Model file for the job. Use its own axes, mm. Face numbers are marked on the shaded views. Give positions to 0.01 mm unless a question says otherwise; leave off trailing zeros. Write each loop counter-clockwise with the first axis right and the second up, starting at its lowest first coordinate (ties: lowest second). Pieces come first, ordered by that corner, then holes. Notation, with made-up numbers: (39.5, -28) - (85.5, -28) arc R32 cw to (85.5, 11) - close; hole circle Ø4 at (20, 45). An arc over 180 degrees is marked (long way). One line per item, written item: value. Start each with the question number.
(1) Drop a flat-ended pin along its axis: P1, Ø4, axis at x = -4, z = 1, coming from the +Y side. Give the stop position or say it passes through.
(2) Cut at A-A, the plane y = 38. List the corners of the cut face in (x, z), and give its area (3 significant figures).
(3) Cut at C-C, the plane x = -8.25. List the corners of the cut face in (y, z).
(4) Cut at B-B, the plane z = -2. List the corners of the cut face in (x, y), and give its area (3 significant figures).
(5) Cut at D-D, the plane y = 8.5. List the corners of the cut face in (x, z), and give its area (3 significant figures).
(6) Mould opens along X. For the marked faces 1, 2 and 3 say: pulls with the +X half, pulls with the -X half, needs draft (parallel to the pull), parting line crosses it, or undercut.
(7) Probe L1, parallel to Z at x = -0.25, y = 20; L2, parallel to X at y = 19, z = -0.5; L3, parallel to X at y = 9, z = -2. List the from-to ranges inside material, lowest first.
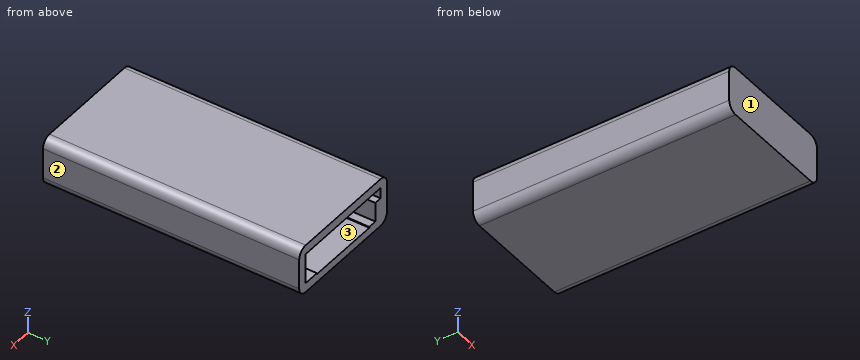
from build123d import *

# Parameters (mm, degrees)
SKETCH1_W           = 20.3
SKETCH1_H           = 7.9
SKETCH1_W_2         = 17.3
SKETCH1_H_2         = 4.9
BOSS_EXTRUDE1_DEPTH = 41.5
SKETCH2_W           = 20.3
SKETCH2_H           = 7.9
BOSS_EXTRUDE2_DEPTH = 1.5
SKETCH3_W           = 1.2
SKETCH3_H           = 3.15
BOSS_EXTRUDE3_DEPTH = 40
SKETCH4_W           = 1.2
SKETCH4_H           = 3.15
BOSS_EXTRUDE4_DEPTH = 17
SKETCH5_W           = 12.1
SKETCH5_H           = 0.3
CUT_EXTRUDE1_DEPTH  = 4.3
FILLET1_R           = 1.5


with BuildPart() as part:
    # Sketch1 → Boss-Extrude1 (new body)
    with BuildSketch(Plane(origin=(0, 0, 0), x_dir=(1, 0, 0), z_dir=(0, 1, 0))):
        Rectangle(SKETCH1_W, SKETCH1_H)
        Rectangle(SKETCH1_W_2, SKETCH1_H_2, mode=Mode.SUBTRACT)
    extrude(amount=BOSS_EXTRUDE1_DEPTH)

    # Sketch2 → Boss-Extrude2 (add)
    with BuildSketch(Plane.XZ):
        Rectangle(SKETCH2_W, SKETCH2_H)
    extrude(amount=-BOSS_EXTRUDE2_DEPTH)

    # Sketch3 → Boss-Extrude3 (add)
    with BuildSketch(Plane(origin=(0, 1.5, 0), x_dir=(1, 0, 0), z_dir=(0, 1, 0))):
        with Locations((-8.05, 0.875)):
            Rectangle(SKETCH3_W, SKETCH3_H)
    extrude(amount=BOSS_EXTRUDE3_DEPTH)

    # Sketch4 → Boss-Extrude4 (add)
    with BuildSketch(Plane(origin=(0, 1.5, 0), x_dir=(1, 0, 0), z_dir=(0, 1, 0))):
        with Locations((8.05, 0.875)):
            Rectangle(SKETCH4_W, SKETCH4_H)
    extrude(amount=BOSS_EXTRUDE4_DEPTH)

    # Sketch5 → Cut-Extrude1 (cut)
    with BuildSketch(Plane(origin=(0, 41.5, 0), x_dir=(1, 0, 0), z_dir=(0, 1, 0))):
        with Locations((0, 2.45)):
            Rectangle(SKETCH5_W, SKETCH5_H)
    extrude(amount=-CUT_EXTRUDE1_DEPTH, mode=Mode.SUBTRACT)

    # Fillet1
    fillet1_edges = [part.edges().sort_by_distance(p)[0] for p in [
        (-10.15, 20.75, 3.95),
        (-10.15, 20.75, -3.95),
        (10.15, 20.75, -3.95),
        (10.15, 20.75, 3.95),
    ]]
    fillet(fillet1_edges, radius=FILLET1_R)


solid = part.part
Answers follow:
1. P1: stops at y = 41.5
2. outline: (-10.15, -2.45) arc R1.5 ccw to (-8.65, -3.95) - (8.65, -3.95) arc R1.5 ccw to (10.15, -2.45) - (10.15, 2.45) arc R1.5 ccw to (8.65, 3.95) - (-8.65, 3.95) arc R1.5 ccw to (-10.15, 2.45) - close; hole (-8.65, 0.7) - (-7.45, 0.7) - (-7.45, -2.45) - (-6.05, -2.45) - (-6.05, -2.6) - (6.05, -2.6) - (6.05, -2.45) - (8.65, -2.45) - (8.65, 2.45) - (-8.65, 2.45) - close
2. area: 75.6 mm²
3. outline: (0, -3.95) - (41.5, -3.95) - (41.5, 0.7) - (1.5, 0.7) - (1.5, 2.45) - (41.5, 2.45) - (41.5, 3.95) - (0, 3.95) - close
4. outline: (-10.15, 0) - (10.15, 0) - (10.15, 41.5) - (8.65, 41.5) - (8.65, 18.5) - (7.45, 18.5) - (7.45, 1.5) - (-7.45, 1.5) - (-7.45, 41.5) - (-10.15, 41.5) - close
4. area: 219 mm²
5. outline: (-10.15, -2.45) arc R1.5 ccw to (-8.65, -3.95) - (8.65, -3.95) arc R1.5 ccw to (10.15, -2.45) - (10.15, 2.45) arc R1.5 ccw to (8.65, 3.95) - (-8.65, 3.95) arc R1.5 ccw to (-10.15, 2.45) - close; hole (-8.65, 0.7) - (-7.45, 0.7) - (-7.45, -2.45) - (7.45, -2.45) - (7.45, 0.7) - (8.65, 0.7) - (8.65, 2.45) - (-8.65, 2.45) - close
5. area: 81.2 mm²
6. face 1: needs draft
6. face 2: pulls with the +X half
6. face 3: undercut
7. L1: z = -3.95 to -2.45, 2.45 to 3.95
7. L2: x = -10.15 to -7.45, 8.65 to 10.15
7. L3: x = -10.15 to -7.45, 7.45 to 10.15
